For this review, take the finished solid that the model builds, in its own axes (mm). Give positions to 0.01 mm unless a question says otherwise; leave off trailing zeros. Loops run counter-clockwise (first coordinate to the right, second up) from the corner with the lowest first, then second, coordinate; pieces in that order, holes last.
```python
from build123d import *

# Parameters (mm, degrees)
EXTRUDE1_DEPTH            = 18.7198
SKETCH13_W                = 30.336118919
SKETCH13_H                = 26.43936277
EXTRUDE2_DEPTH            = 40.057833358
F_6_32_TAPPED_HOLE2_D     = 2.7051
EXTRUDE3_DEPTH            = 40.057833358
F_6_32_TAPPED_HOLE1_D     = 2.7051
F_8_32_TAPPED_HOLE5_D     = 3.4544
F_8_32_TAPPED_HOLE5_DEPTH = 19.05
F_8_32_TAPPED_HOLE5_TIP   = 1.037806461
SKETCH22_W                = 9.398
SKETCH22_H                = 21.690053411
EXTRUDE4_DEPTH            = 33.232321948
CHAMFER1_SIZE             = 5.588
CUT_EXTRUDE1_DEPTH        = 33.232321948


with BuildPart() as part:
    # Sketch1 → Extrude1 (new body)
    with BuildSketch(Plane.XY):
        with BuildLine():
            Line((0, 0), (0, -13.17458008))
            Line((0, -13.17458008), (15.324208221, -28.498788301))
            ThreePointArc((15.324208221, -28.498788301), (19.05, -6.58729004), (15.324208221, 15.324208221))
            Line((15.324208221, 15.324208221), (0, 15.324208221))
            Line((0, 15.324208221), (0, 0))
        make_face()
    extrude(amount=EXTRUDE1_DEPTH)

    # Sketch13 → Extrude2 (cut, through all)
    with BuildSketch(Plane.XY.offset(18.7198)):
        with Locations((15.16805946, 17.825101305)):
            Rectangle(SKETCH13_W, SKETCH13_H)
    extrude(amount=-EXTRUDE2_DEPTH, mode=Mode.SUBTRACT)

    # #6-32 Tapped Hole2 (through all)
    with Locations(Plane.XY.offset(18.7198)):
        with Locations((13.6525, -1.50729004)):
            Hole(F_6_32_TAPPED_HOLE2_D / 2)

    # Sketch14 → Extrude3 (cut, through all)
    with BuildSketch(Plane.XY.offset(18.7198)):
        Polygon((0.684709755, -13.859289835), (7.276217748, -7.267781842), (18.052525094, -18.044089188), (21.915716214, -21.907280308), (15.324208221, -28.498788301), align=None)
    extrude(amount=-EXTRUDE3_DEPTH, mode=Mode.SUBTRACT)

    # #6-32 Tapped Hole1 (through all)
    with Locations(Plane(origin=(12.651735758, -12.643299852, 14.4399), x_dir=(-0.707106781187, 0.707106781187, 0), z_dir=(-0.707106781187, -0.707106781187, 0))):
        with Locations((0, 0), (0, 10.16)):
            Hole(F_6_32_TAPPED_HOLE1_D / 2)

    # #8-32 Tapped Hole5
    with Locations(Plane.ZY):
        with Locations((9.3599, -6.58729004)):
            Hole(F_8_32_TAPPED_HOLE5_D / 2, depth=F_8_32_TAPPED_HOLE5_DEPTH)
            with Locations((0, 0, -(F_8_32_TAPPED_HOLE5_DEPTH + F_8_32_TAPPED_HOLE5_TIP / 2))):  # 118° drill point
                Cone(0, F_8_32_TAPPED_HOLE5_D / 2, F_8_32_TAPPED_HOLE5_TIP, mode=Mode.SUBTRACT)

    # Sketch22 → Extrude4 (cut, through all)
    with BuildSketch(Plane.XY.offset(18.7198)):
        with Locations((4.699, -6.239606786)):
            Rectangle(SKETCH22_W, SKETCH22_H)
    extrude(amount=-EXTRUDE4_DEPTH, mode=Mode.SUBTRACT)

    # Chamfer1
    chamfer1_edges = [part.edges().sort_by_distance(p)[0] for p in [
        (9.398, 4.60541992, 9.3599),
    ]]
    chamfer(chamfer1_edges, length=CHAMFER1_SIZE)

    # Sketch27 → Cut-Extrude1 (cut, through all)
    with BuildSketch(Plane.XY.offset(18.7198)):
        Polygon((17.154499481, -17.146063576), (21.888027801, -12.412535256), (22.786053413, -13.310560868), (18.052525094, -18.044089188), align=None)
    extrude(amount=-CUT_EXTRUDE1_DEPTH, mode=Mode.SUBTRACT)


solid = part.part
```
Q1. For pin 1 Ø2 at (y, z) = (-10, 16) entering from +X, flat-tipped, find the tip position at first contact; note if it passes through.
Answers:
pin 1: stops at x = 19.01
Q2. For probe 1 along Z at (x, y) = (16, -8); probe 2 along Z at (x, y) = (18, -6.5); probe 3 along Z at (x, y) = (16.25, -10.25), list the stretches that pass through material, from the lowest coordinate up.
Answers:
probe 1: z = 0 to 3.28, 5.28 to 8.37, 10.35 to 13.44, 15.44 to 18.72
probe 2: z = 0 to 3.05, 5.51 to 7.63, 11.08 to 13.21, 15.67 to 18.72
probe 3: z = 0 to 3.23, 5.33 to 13.39, 15.49 to 18.72
Q3. Consider section B-B on x = 13.25. Count the separate pieces of the cut face and the enclosed holes in it, plus the area to 3 significant figures.
Answers:
separate pieces: 2
enclosed holes: 1
area: 230 mm2
Q4. Consider section A-A on z = 8. Give the boundary of the cut face in (x, y).
Answers:
outline: (9.4, -9.39) - (17.15, -17.15) - (18.39, -15.91) arc R66.29 ccw to (19.04, -7.65) - (9.4, -7.65) - close; (9.4, -5.52) - (19.04, -5.52) arc R66.29 ccw to (18.1, 4.61) - (14.99, 4.61) - (9.4, -0.98) - close; hole circle Ø2.71 at (13.65, -1.51)
Q5. Mouldability with a two-part tool opening along Z and no side actions: class faces 1 (the cylindrical face through (14.593, -8.791, 14.38)), 2 (the flat face through (15, -6, 18.72)), 3 (the cylindrical face through (12.362, -1.101, 9.229)) as +Z half, -Z half, draft (parallel to the pull), parting line (faces both ways), or undercut.
Answers:
face 1: undercut
face 2: +Z half
face 3: draft
Q6. Consider section D-D on z = 17. Give the boundary of the cut face in (x, y).
Answers:
outline: (9.4, -9.39) - (17.15, -17.15) - (18.39, -15.91) arc R66.29 ccw to (18.1, 4.61) - (14.99, 4.61) - (9.4, -0.98) - close; hole circle Ø2.71 at (13.65, -1.51)
Q7. Consider section C-C on z = 5. Give the boundary of the cut face in (x, y).
Answers:
outline: (9.4, -9.39) - (11.84, -11.83) - (19.02, -4.65) arc R66.29 ccw to (18.1, 4.61) - (14.99, 4.61) - (9.4, -0.98) - close; (13.46, -13.45) - (17.15, -17.15) - (18.39, -15.91) arc R66.29 ccw to (19.04, -7.88) - close; hole circle Ø2.71 at (13.65, -1.51)
